Could you check a few things on this drawing? It's one solid part, dimensions in mm from its lowest x, y, z. Round coordinates to 2 decimals unless told otherwise and drop trailing zeros. Write each loop counter-clockwise with the first axis right and the second up, starting at its lowest first coordinate (ties: lowest second). Pieces come first, ordered by that corner, then holes. Notation, with made-up numbers: M 10.5,22.25 L 61.5,22.25 A14 ccw 61.5,31.25 Z; hole C -19.75,6 d11. An arc over 180 degrees is marked long. One line per item, written item: value. Start each with the question number.
(1) I want a section at D-D on z = 29.25. Please give me the cut outline in (x, y), and give its area (3 significant figures).
(2) I want a section at B-B on x = 21. Please give me the cut outline in (y, z).
(3) I want a section at A-A on z = 21. Please give me the cut outline in (x, y), and give its area (3 significant figures).
(4) I'm going to push flat-ended pins straight in: pin 1 Ø1.5 at (y, z) = (1.5, 26) entering from +X (1 decimal); pin 2 Ø1.5 at (x, y) = (26.5, 1.5) entering from -Z. Where does each tip first touch, or does it pass through?
(5) Thinking about a two-plate mould opening in Z: for the marked faces 1, 2 and 3, which applies, released by +Z, released by -Z, zero draft, split by the parting line, or undercut?
(6) If I drill on L1, parallel to Z at x = 21, y = 0.45; L2, parallel to Z at x = 21, y = 5.55; L3, parallel to Z at x = 6, y = 6, over which ranges is the centre line in solid material (lowest first)?
(7) I want a section at C-C on y = 2. Please give me the cut outline in (x, z), and give its area (3 significant figures).
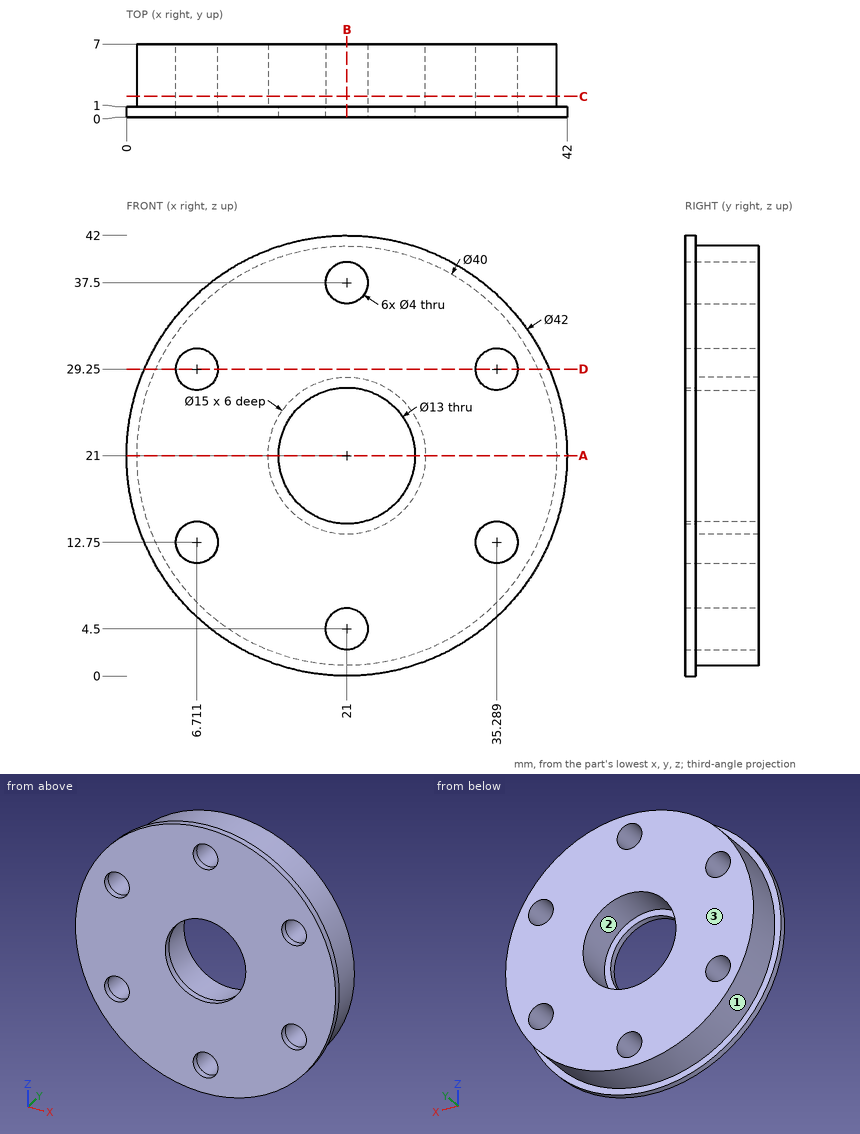
Found:
1. outline: M 1.69,0 L 4.71,0 L 4.71,7 L 2.78,7 L 2.78,1 L 1.69,1 Z; M 8.71,0 L 33.29,0 L 33.29,7 L 8.71,7 Z; M 37.29,0 L 40.31,0 L 40.31,1 L 39.22,1 L 39.22,7 L 37.29,7 Z
1. area: 201 mm²
2. outline: M 0,0 L 1,0 L 1,1 L 7,1 L 7,2.5 L 0,2.5 Z; M 0,6.5 L 7,6.5 L 7,13.5 L 1,13.5 L 1,14.5 L 0,14.5 Z; M 0,27.5 L 1,27.5 L 1,28.5 L 7,28.5 L 7,35.5 L 0,35.5 Z; M 0,39.5 L 7,39.5 L 7,41 L 1,41 L 1,42 L 0,42 Z
3. outline: M 0,0 L 14.5,0 L 14.5,1 L 13.5,1 L 13.5,7 L 1,7 L 1,1 L 0,1 Z; M 27.5,0 L 42,0 L 42,1 L 41,1 L 41,7 L 28.5,7 L 28.5,1 L 27.5,1 Z
3. area: 179 mm²
4. pin 1: stops at x = 41.5
4. pin 2: stops at z = 0.59
5. face 1: split by the parting line
5. face 2: undercut
5. face 3: zero draft
6. L1: z = 0 to 2.5, 6.5 to 14.5, 27.5 to 35.5, 39.5 to 42
6. L2: z = 1 to 2.5, 6.5 to 13.5, 28.5 to 35.5, 39.5 to 41
6. L3: z = 7.77 to 10.88, 14.62 to 27.38, 31.12 to 34.23
7. outline: C 21,21 d40; hole C 6.71,12.75 d4; hole C 6.71,29.25 d4; hole C 21,21 d15; hole C 21,4.5 d4; hole C 21,37.5 d4; hole C 35.29,12.75 d4; hole C 35.29,29.25 d4
7. area: 1,000 mm²
